Geometry: final body of the model. Coordinates: model frame, mm. Face numbers are marked on the shaded views. A direction names the side the tool comes from. Give positions to 0.01 mm unless a question says otherwise; leave off trailing zeros. Order: outer loops, then holes, each group sorted by start corner. A loop starts at its lowest first (then second) coordinate and runs counter-clockwise, first axis right, second up. Notation, with made-up numbers: (79.25, -30) - (83.25, -30) arc R17 ccw to (83.25, -22) - close; hole circle Ø3 at (66, 89). An arc over 180 degrees is marked (long way). Use one line per item in the form item = value.
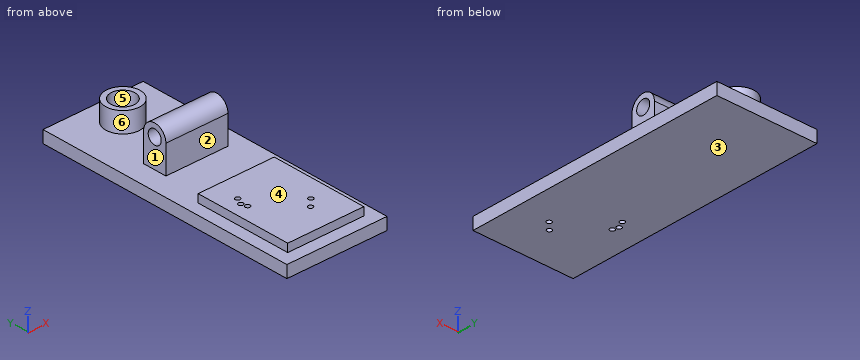
from build123d import *

# Parameters (mm, degrees)
F0_W      = 5.4119601846
F0_H      = 3
F0_W_2    = 25
F0_H_2    = 35.3582080007
F0_R      = 4.2675896262
F0_W_3    = 4.1414871812
F0_W_4    = 3.0508699417
F0_W_5    = 6.3956826925
F0_W_6    = 19
F0_H_3    = 13.8665742949
F0_R_2    = 0.6
F1_DEPTH  = 3
F2_DEPTH  = 2
F0_R_3    = 3
F3_DEPTH  = 5
F4_DEPTH  = 3
F8_DEPTH  = 15.5
F9_W      = 25
F9_H      = 65.3582080007
F9_R      = 1.5
F9_R_2    = 0.6
F10_DEPTH = 3


with BuildPart() as f1:
    # F0 (on Top) → F1 (new body)
    with BuildSketch(Plane.XY):
        with Locations((-13.243149966, -1.5)):
            Rectangle(F0_W, F0_H)
        with Locations((-9.5, 44.6791040003)):
            Rectangle(F0_W_2, F0_H_2)
        with Locations((-9.5, 54.3582080007)):
            Circle(F0_R, mode=Mode.SUBTRACT)
        with Locations((-2.0707435906, -1.5)):
            Rectangle(F0_W_3, F0_H)
        with Locations((-17.4745650291, -1.5)):
            Rectangle(F0_W_4, F0_H)
        with Locations((-7.3393285275, -1.5)):
            Rectangle(F0_W_5, F0_H)
        Polygon((0, 10.1334257051), (0, 0), (0, -3), (3, -3), (3, 27), (-22, 27), (-22, -3), (-19, -3), (-19, 0), (-19, 10.1334257051), (-19, 24), (0, 24), align=None)
        with Locations((-9.5, 17.0667128526)):
            Rectangle(F0_W_6, F0_H_3)
        with Locations((-15.8, 16)):
            Circle(F0_R_2, mode=Mode.SUBTRACT)
        with Locations((-15.4, 14.6)):
            Circle(F0_R_2, mode=Mode.SUBTRACT)
        with Locations((-14.9, 17.8)):
            Circle(F0_R_2, mode=Mode.SUBTRACT)
        Polygon((-4.1414871812, 0), (0, 0), (0, 10.1334257051), (-19, 10.1334257051), (-19, 0), (-15.9491300583, 0), (-10.5371698737, 0), align=None)
        with Locations((-7.14, 6.6)):
            Circle(F0_R_2, mode=Mode.SUBTRACT)
        with Locations((-5.1, 8.7)):
            Circle(F0_R_2, mode=Mode.SUBTRACT)
    extrude(amount=-F1_DEPTH)

    # F0 (on Top) → F2 (join)
    with BuildSketch(Plane.XY):
        with Locations((-9.5, 17.0667128526)):
            Rectangle(F0_W_6, F0_H_3)
        with Locations((-15.8, 16)):
            Circle(F0_R_2, mode=Mode.SUBTRACT)
        with Locations((-15.4, 14.6)):
            Circle(F0_R_2, mode=Mode.SUBTRACT)
        with Locations((-14.9, 17.8)):
            Circle(F0_R_2, mode=Mode.SUBTRACT)
        Polygon((-4.1414871812, 0), (0, 0), (0, 10.1334257051), (-19, 10.1334257051), (-19, 0), (-15.9491300583, 0), (-10.5371698737, 0), align=None)
        with Locations((-7.14, 6.6)):
            Circle(F0_R_2, mode=Mode.SUBTRACT)
        with Locations((-5.1, 8.7)):
            Circle(F0_R_2, mode=Mode.SUBTRACT)
    extrude(amount=F2_DEPTH)

    # F0 (on Top) → F3 (join)
    with BuildSketch(Plane.XY):
        with Locations((-9.5, 54.3582080007)):
            Circle(F0_R)
        with Locations((-9.5, 54.3582080007)):
            Circle(F0_R_3, mode=Mode.SUBTRACT)
    extrude(amount=F3_DEPTH)

    # F0 (on Top) → F4 (join)
    with BuildSketch(Plane.XY):
        with Locations((-9.5, 54.3582080007)):
            Circle(F0_R)
        with Locations((-9.5, 54.3582080007)):
            Circle(F0_R_3, mode=Mode.SUBTRACT)
        with Locations((-9.5, 54.3582080007)):
            Circle(F0_R_3)
    extrude(amount=-F4_DEPTH)

    # F7 (on offset) → F8 (join)
    with BuildSketch(Plane(origin=(-16.8, 0, 0), x_dir=(0, -1, 0), z_dir=(-1, 0, 0))):
        with BuildLine():
            ThreePointArc((-35, 7), (-38, 10), (-41, 7))
            Line((-41, 7), (-39.75, 7))
            ThreePointArc((-39.75, 7), (-38, 8.75), (-36.25, 7))
            Line((-36.25, 7), (-35, 7))
        make_face()
        with BuildLine():
            Line((-41, 7), (-41, 0))
            Line((-41, 0), (-35, 0))
            Line((-35, 0), (-35, 7))
            Line((-35, 7), (-36.25, 7))
            ThreePointArc((-36.25, 7), (-38, 5.25), (-39.75, 7))
            Line((-39.75, 7), (-41, 7))
        make_face()
    extrude(amount=-F8_DEPTH)

    # F9 (on face) → F10 (join)
    with BuildSketch(Plane(origin=(0, 0, -3), x_dir=(1, 0, 0), z_dir=(0, 0, -1))):
        with Locations((-9.5, -29.6791040003)):
            Rectangle(F9_W, F9_H)
        with Locations((-9.5, -54.3582080007)):
            Circle(F9_R, mode=Mode.SUBTRACT)
        with Locations((-15.8, -16)):
            Circle(F9_R_2, mode=Mode.SUBTRACT)
        with Locations((-14.9, -17.8)):
            Circle(F9_R_2, mode=Mode.SUBTRACT)
        with Locations((-15.4, -14.6)):
            Circle(F9_R_2, mode=Mode.SUBTRACT)
        with Locations((-7.14, -6.6)):
            Circle(F9_R_2, mode=Mode.SUBTRACT)
        with Locations((-5.1, -8.7)):
            Circle(F9_R_2, mode=Mode.SUBTRACT)
    extrude(amount=-F10_DEPTH)


solid = f1.part
(1) Cut plane A-A on y = 17.8. Output: boundary loops of the cut face in (x, z).
Computed values:
outline = (-22, -3) - (-15.5, -3) - (-15.5, 2) - (-19, 2) - (-19, 0) - (-22, 0) - close; (-14.3, -3) - (3, -3) - (3, 0) - (0, 0) - (0, 2) - (-14.3, 2) - close
(2) Cut plane C-C on z = 1. Give the number of separate pieces and of enclosed holes in the cut face, plus the area to 3 significant figures.
Computed values:
separate_pieces = 3
enclosed_holes = 6
area = 572 mm²
(3) Contact query for flat-ended pins moving along their axis: pin 1 Ø9.5 at (x, y) = (-11.5, 17) entering from +Z; pin 2 Ø1.5 at (x, y) = (-7, 55) entering from +Z; pin 3 Ø2 at (x, z) = (-8.5, 2) entering from +Y. Output: stop coordinate, or through.
Computed values:
pin_1 = 2
pin_2 = 5
pin_3 = 58.63
(4) Ray query, line 1 along Y through (x, z) = (-9.75, 1); line 2 along Y through (x, z) = (-12, 4.5); line 3 along Z through (x, y) = (-8.25, 38). Return the intervals inside material, ascending.
Computed values:
line_1 = 0 to 24, 35 to 41, 50.1 to 51.37, 57.35 to 58.62
line_2 = 35 to 41, 50.9 to 52.7, 56.02 to 57.82
line_3 = -3 to 5.25, 8.75 to 10
(5) Cut plane D-D on x = -18.25. Output: boundary loops of the cut face in (y, z).
Computed values:
outline = (-3, -3) - (62.36, -3) - (62.36, 0) - (24, 0) - (24, 2) - (0, 2) - (0, 0) - (-3, 0) - close
(6) Reachability of the marked faces 1, 2 and 3 from +Z, -Z, +X, -X, +Y, -Y: full face, straight path, thin tool, end or side. Return the list, or none.
Computed values:
face_1 = +Z, -X, +Y
face_2 = +Z, +X, -X
face_3 = -Z, +X, -X, +Y, -Y
(7) Cut plane B-B on x = -7.14. Output: boundary loops of the cut face in (y, z).
Computed values:
outline = (-3, -3) - (6, -3) - (6, 2) - (0, 2) - (0, 0) - (-3, 0) - close; (7.2, -3) - (62.36, -3) - (62.36, 0) - (57.91, 0) - (57.91, 5) - (56.21, 5) - (56.21, 0) - (52.51, 0) - (52.51, 5) - (50.8, 5) - (50.8, 0) - (41, 0) - (41, 7) arc R3 ccw to (35, 7) - (35, 0) - (24, 0) - (24, 2) - (7.2, 2) - close; hole circle Ø3.5 at (38, 7)
(8) Pull-direction query (X, two-part tool) for the marked faces 4, 5 and 6; classes: released by +X, released by -X, zero draft, split by the parting line, or undercut.
Computed values:
face_4 = zero draft
face_5 = undercut
face_6 = split by the parting line
